Can you work these out from the model? Positions are in its coordinate system, mm. A direction names the side the tool comes from. Give positions to 0.01 mm unless a question says otherwise; leave off trailing zeros. Write each loop counter-clockwise with the first axis right and the second up, starting at its lowest first coordinate (ties: lowest second). Pieces come first, ordered by that corner, then holes.
from build123d import *

# Parameters (mm, degrees)
F1_DEPTH = 228.6


with BuildPart() as f1:
    # F0 (on Right) → F1 (new body)
    with BuildSketch(Plane.YZ):
        with BuildLine():
            Line((-20.088481, -9.788837), (-20.088481, -10.288837))
            Line((-20.088481, -10.288837), (-21.28859, -10.288837))
            ThreePointArc((-21.28859, -10.288837), (-21.500722, -10.376705), (-21.58859, -10.588837))
            Line((-21.58859, -10.588837), (-21.58859, -23.988949))
            ThreePointArc((-21.58859, -23.988949), (-20.70991, -26.11027), (-18.58859, -26.988949))
            Line((-18.58859, -26.988949), (-5.188544, -26.988949))
            ThreePointArc((-5.188544, -26.988949), (-4.976411, -26.901081), (-4.888544, -26.688949))
            Line((-4.888544, -26.688949), (-4.888544, -25.488841))
            Line((-4.888544, -25.488841), (-4.388544, -25.488841))
            ThreePointArc((-4.388544, -25.488841), (-4.176411, -25.400973), (-4.088544, -25.188841))
            Line((-4.088544, -25.188841), (-4.088544, -21.288841))
            ThreePointArc((-4.088544, -21.288841), (-4.176411, -21.076709), (-4.388544, -20.988841))
            Line((-4.388544, -20.988841), (-9.138663, -20.988841))
            Line((-9.138663, -20.988841), (-9.138663, -16.881665))
            Line((-9.138663, -16.881665), (-6.245729, -13.988731))
            Line((-6.245729, -13.988731), (-2.211433, -13.988731))
            ThreePointArc((-2.211433, -13.988731), (-0.669869, -14.363044), (0.91149, -14.48887))
            Line((0.91149, -14.48887), (0.91149, -4.48887))
            Line((0.91149, -4.48887), (-9.08851, -4.48887))
            ThreePointArc((-9.08851, -4.48887), (-8.962684, -6.070229), (-8.588371, -7.611793))
            Line((-8.588371, -7.611793), (-8.588371, -11.646022))
            Line((-8.588371, -11.646022), (-11.481305, -14.538956))
            Line((-11.481305, -14.538956), (-15.588481, -14.538956))
            Line((-15.588481, -14.538956), (-15.588481, -9.788837))
            ThreePointArc((-15.588481, -9.788837), (-15.676349, -9.576705), (-15.888481, -9.488837))
            Line((-15.888481, -9.488837), (-19.788481, -9.488837))
            ThreePointArc((-19.788481, -9.488837), (-20.000613, -9.576705), (-20.088481, -9.788837))
        make_face()
        with BuildLine():
            ThreePointArc((-8.588371, -1.365947), (-8.962684, -2.907511), (-9.08851, -4.48887))
            Line((-9.08851, -4.48887), (0.91149, -4.48887))
            Line((0.91149, -4.48887), (0.91149, 5.51113))
            ThreePointArc((0.91149, 5.51113), (-0.669869, 5.385303), (-2.211433, 5.010991))
            Line((-2.211433, 5.010991), (-6.245729, 5.010991))
            Line((-6.245729, 5.010991), (-9.138663, 7.903925))
            Line((-9.138663, 7.903925), (-9.138663, 12.011101))
            Line((-9.138663, 12.011101), (-4.388544, 12.011101))
            ThreePointArc((-4.388544, 12.011101), (-4.176411, 12.098969), (-4.088544, 12.311101))
            Line((-4.088544, 12.311101), (-4.088544, 16.211101))
            ThreePointArc((-4.088544, 16.211101), (-4.176411, 16.423233), (-4.388544, 16.511101))
            Line((-4.388544, 16.511101), (-4.888544, 16.511101))
            Line((-4.888544, 16.511101), (-4.888544, 17.711209))
            ThreePointArc((-4.888544, 17.711209), (-4.976411, 17.923341), (-5.188544, 18.011209))
            Line((-5.188544, 18.011209), (-18.58859, 18.011209))
            ThreePointArc((-18.58859, 18.011209), (-20.70991, 17.13253), (-21.58859, 15.011209))
            Line((-21.58859, 15.011209), (-21.58859, 1.611097))
            ThreePointArc((-21.58859, 1.611097), (-21.500722, 1.398965), (-21.28859, 1.311097))
            Line((-21.28859, 1.311097), (-20.088481, 1.311097))
            Line((-20.088481, 1.311097), (-20.088481, 0.811097))
            ThreePointArc((-20.088481, 0.811097), (-20.000613, 0.598965), (-19.788481, 0.511097))
            Line((-19.788481, 0.511097), (-15.888481, 0.511097))
            ThreePointArc((-15.888481, 0.511097), (-15.676349, 0.598965), (-15.588481, 0.811097))
            Line((-15.588481, 0.811097), (-15.588481, 5.561216))
            Line((-15.588481, 5.561216), (-11.481305, 5.561216))
            Line((-11.481305, 5.561216), (-8.588371, 2.668282))
            Line((-8.588371, 2.668282), (-8.588371, -1.365947))
        make_face()
        with BuildLine():
            Line((0.91149, 5.51113), (0.91149, -4.48887))
            Line((0.91149, -4.48887), (10.91149, -4.48887))
            ThreePointArc((10.91149, -4.48887), (10.785663, -2.907511), (10.41135, -1.365947))
            Line((10.41135, -1.365947), (10.41135, 2.668282))
            Line((10.41135, 2.668282), (13.304285, 5.561216))
            Line((13.304285, 5.561216), (14.016842, 5.561216))
            Line((14.016842, 5.561216), (17.41146, 5.561216))
            Line((17.41146, 5.561216), (17.41146, 0.811097))
            ThreePointArc((17.41146, 0.811097), (17.499328, 0.598965), (17.71146, 0.511097))
            Line((17.71146, 0.511097), (21.61146, 0.511097))
            ThreePointArc((21.61146, 0.511097), (21.823593, 0.598965), (21.91146, 0.811097))
            Line((21.91146, 0.811097), (21.91146, 1.311097))
            Line((21.91146, 1.311097), (23.111569, 1.311097))
            ThreePointArc((23.111569, 1.311097), (23.323701, 1.398965), (23.411569, 1.611097))
            Line((23.411569, 1.611097), (23.411569, 15.011209))
            ThreePointArc((23.411569, 15.011209), (22.532889, 17.13253), (20.411569, 18.011209))
            Line((20.411569, 18.011209), (7.011523, 18.011209))
            ThreePointArc((7.011523, 18.011209), (6.799391, 17.923341), (6.711523, 17.711209))
            Line((6.711523, 17.711209), (6.711523, 16.511101))
            Line((6.711523, 16.511101), (6.211523, 16.511101))
            ThreePointArc((6.211523, 16.511101), (5.999391, 16.423233), (5.911523, 16.211101))
            Line((5.911523, 16.211101), (5.911523, 12.311101))
            ThreePointArc((5.911523, 12.311101), (5.999391, 12.098969), (6.211523, 12.011101))
            Line((6.211523, 12.011101), (10.961642, 12.011101))
            Line((10.961642, 12.011101), (10.961642, 7.903925))
            Line((10.961642, 7.903925), (8.068708, 5.010991))
            Line((8.068708, 5.010991), (4.034413, 5.010991))
            ThreePointArc((4.034413, 5.010991), (2.492849, 5.385303), (0.91149, 5.51113))
        make_face()
        with BuildLine():
            Line((10.91149, -4.48887), (0.91149, -4.48887))
            Line((0.91149, -4.48887), (0.91149, -14.48887))
            ThreePointArc((0.91149, -14.48887), (2.492849, -14.363044), (4.034413, -13.988731))
            Line((4.034413, -13.988731), (8.068708, -13.988731))
            Line((8.068708, -13.988731), (10.961642, -16.881665))
            Line((10.961642, -16.881665), (10.961642, -20.988841))
            Line((10.961642, -20.988841), (6.211523, -20.988841))
            ThreePointArc((6.211523, -20.988841), (5.999391, -21.076709), (5.911523, -21.288841))
            Line((5.911523, -21.288841), (5.911523, -25.188841))
            ThreePointArc((5.911523, -25.188841), (5.999391, -25.400973), (6.211523, -25.488841))
            Line((6.211523, -25.488841), (6.711523, -25.488841))
            Line((6.711523, -25.488841), (6.711523, -26.688949))
            ThreePointArc((6.711523, -26.688949), (6.799391, -26.901081), (7.011523, -26.988949))
            Line((7.011523, -26.988949), (20.411569, -26.988949))
            ThreePointArc((20.411569, -26.988949), (22.532889, -26.11027), (23.411569, -23.988949))
            Line((23.411569, -23.988949), (23.411569, -10.588837))
            ThreePointArc((23.411569, -10.588837), (23.323701, -10.376705), (23.111569, -10.288837))
            Line((23.111569, -10.288837), (21.91146, -10.288837))
            Line((21.91146, -10.288837), (21.91146, -9.788837))
            ThreePointArc((21.91146, -9.788837), (21.823593, -9.576705), (21.61146, -9.488837))
            Line((21.61146, -9.488837), (17.71146, -9.488837))
            ThreePointArc((17.71146, -9.488837), (17.499328, -9.576705), (17.41146, -9.788837))
            Line((17.41146, -9.788837), (17.41146, -14.538956))
            Line((17.41146, -14.538956), (13.304285, -14.538956))
            Line((13.304285, -14.538956), (10.41135, -11.646022))
            Line((10.41135, -11.646022), (10.41135, -7.611793))
            ThreePointArc((10.41135, -7.611793), (10.785663, -6.070229), (10.91149, -4.48887))
        make_face()
    extrude(amount=F1_DEPTH)


solid = f1.part
(1) Will these pins go through, and if not, where does the flat tip stop? P1, Ø1.2, axis at x = 97, z = -10, coming from the +Y side; P2, Ø1, axis at x = 165.5, z = 17, coming from the -Y side; P3, Ø2, axis at x = 154.5, y = -1.5, coming from the +Z side; P4, Ø1, axis at x = 83.5, y = 22.5, coming from the -Z side.
Returned:
P1: stops at y = 23.41
P2: stops at y = -21.19
P3: stops at z = 5.41
P4: stops at z = -26.53
(2) If I drill on L1, parallel to Z at x = 112.5, y = 7.5; L2, parallel to Z at x = 112, y = -17; L3, parallel to Y at x = 155, z = 13, over which ranges is the centre line in solid material (lowest first)?
Returned:
L1: z = -26.99 to -20.99, -13.99 to 5.01, 12.01 to 18.01
L2: z = -26.99 to -9.49, 0.51 to 18.01
L3: y = -21.59 to -4.09, 5.91 to 23.41
(3) Imagine slicing it at A-A, the plane y = -13.5. Write out the boundary of the cut face in (x, z), plus the area to 3 significant figures.
Returned:
outline: (0, -26.99) - (228.6, -26.99) - (228.6, -14.54) - (0, -14.54) - close; (0, 5.56) - (228.6, 5.56) - (228.6, 18.01) - (0, 18.01) - close
area: 5,690 mm2
(4) If we mould it in two halves opening along Y, with no side actions, what happens to faces 4 (the face through (113, 23.412, 8)), 5 (the face through (113, 10.962, -19)), 6 (the face through (228.6, 1, -4))? For each: +Y half, -Y half, draft (parallel to the pull), parting line (faces both ways), or undercut.
Returned:
face 4: +Y half
face 5: undercut
face 6: draft
(5) For faces 1 (the face through (113, -21.589, -17)), 2 (the face through (113, -14, -14.539)), 3 (the face through (113, -4.089, 14)), which set-ups out of +Z, -Z, +X, -X, +Y, -Y let a thin tool reach every point of the face, with its end or its side?
Returned:
face 1: +Z, -Z, +X, -X, -Y
face 2: +X, -X
face 3: +Z, +X, -X
